from build123d import *

# Parameters (mm, degrees)
SKETCH_1_W          = 45
SKETCH_1_H          = 42
EXTRUDE_1_DEPTH     = 2
SKETCH_2_R          = 11
SKETCH_2_R_2        = 1.5
CUT_EXTRUDE_1_DEPTH = 2
SKETCH_3_W          = 2
SKETCH_3_H          = 42
EXTRUDE_2_DEPTH     = 40
SKETCH_4_R          = 5
SKETCH_4_R_2        = 2.5
EXTRUDE_3_DEPTH     = 10
SKETCH_5_R          = 2
CUT_EXTRUDE_2_DEPTH = 81.950602221


with BuildPart() as part:
    # 草图1 → 凸台-拉伸1 (new body)
    with BuildSketch(Plane(origin=(0, 0, 0), x_dir=(1, 0, 0), z_dir=(0, 1, 0))):
        with Locations((22.5, 21)):
            Rectangle(SKETCH_1_W, SKETCH_1_H)
    extrude(amount=EXTRUDE_1_DEPTH)

    # 草图2 → 切除-拉伸1 (cut)
    with BuildSketch(Plane(origin=(0, 2, 0), x_dir=(1, 0, 0), z_dir=(0, 1, 0))):
        with Locations(Location((21, 21, 0), (0, 0, 270))):
            Circle(SKETCH_2_R)
        with Locations(Location((5.5, 5.5, 0), (0, 0, 270))):
            Circle(SKETCH_2_R_2)
        with Locations(Location((5.5, 36.5, 0), (0, 0, 270))):
            Circle(SKETCH_2_R_2)
        with Locations(Location((36.5, 36.5, 0), (0, 0, 270))):
            Circle(SKETCH_2_R_2)
        with Locations(Location((36.5, 5.5, 0), (0, 0, 270))):
            Circle(SKETCH_2_R_2)
    extrude(amount=-CUT_EXTRUDE_1_DEPTH, mode=Mode.SUBTRACT)

    # 草图3 → 凸台-拉伸2 (add)
    with BuildSketch(Plane(origin=(0, 2, 0), x_dir=(1, 0, 0), z_dir=(0, 1, 0))):
        with Locations((44, 21)):
            Rectangle(SKETCH_3_W, SKETCH_3_H)
    extrude(amount=EXTRUDE_2_DEPTH)

    # 草图4 → 凸台-拉伸3 (add)
    with BuildSketch(Plane(origin=(45, 0, 0), x_dir=(0, 0, -1), z_dir=(1, 0, 0))):
        with Locations(Location((21, 20, 0), (0, 0, 180))):
            Circle(SKETCH_4_R)
        with Locations((21, 20)):
            Circle(SKETCH_4_R_2, mode=Mode.SUBTRACT)
    extrude(amount=EXTRUDE_3_DEPTH)

    # 草图5 → 切除-拉伸2 (cut, through all)
    with BuildSketch(Plane.XY):
        with Locations((50, 20)):
            Circle(SKETCH_5_R)
    extrude(amount=-CUT_EXTRUDE_2_DEPTH, mode=Mode.SUBTRACT)


solid = part.part
Input: part model. Units: mm. Frame: model coordinates. A direction names the side the tool comes from. Give positions to 0.01 mm unless a question says otherwise; leave off trailing zeros. Order: outer loops, then holes, each group sorted by start corner. A loop starts at its lowest first (then second) coordinate and runs counter-clockwise, first axis right, second up. Notation, with made-up numbers: (15, -21) -> (65, -21) arc R19 cw to (65, -12) -> close; hole circle Ø8 at (48.25, -10). An arc over 180 degrees is marked (long way). Use one line per item in the form item = value.
1) Section D-D, the plane z = -17.5. Return loops of the section in (x, y).
Response values:
outline = (0, 0) -> (10.57, 0) -> (10.57, 2) -> (0, 2) -> close; (31.43, 0) -> (45, 0) -> (45, 16.43) -> (55, 16.43) -> (55, 23.57) -> (45, 23.57) -> (45, 42) -> (43, 42) -> (43, 2) -> (31.43, 2) -> close; hole circle Ø4 at (50, 20)
2) Section B-B, the plane z = -5.5. Return loops of the section in (x, y).
Response values:
outline = (0, 0) -> (4, 0) -> (4, 2) -> (0, 2) -> close; (7, 0) -> (35, 0) -> (35, 2) -> (7, 2) -> close; (38, 0) -> (45, 0) -> (45, 42) -> (43, 42) -> (43, 2) -> (38, 2) -> close
3) Mould query, pull axis Z, two halves, no side actions, for faces 4 (the flat face through (32, 1, 0)), 5 (the cylindrical face through (50, 23, -25)), 6 (the cylindrical face through (35.6, 1, -37.7)). Classes: pulls with the +Z half, pulls with the -Z half, needs draft (parallel to the pull), parting line crosses it, or undercut.
Response values:
face_4 = pulls with the +Z half
face_5 = parting line crosses it
face_6 = undercut
4) Line query: probe 1 along X at (y, z) = (1.6, -36.5); probe 2 along X at (y, z) = (20, -18); probe 3 along Y at (x, z) = (37.5, -1.5). Output: solid intervals per line, ascending.
Response values:
probe_1 = 0 to 4, 7 to 35, 38 to 45
probe_2 = 43 to 48, 52 to 55
probe_3 = 0 to 2
5) Reachability of faces 1 (the flat face through (45, 20, -21)), 2 (the flat face through (43, 22, -21)), 3 (the flat face through (44, 42, -21)) from +Z, -Z, +X, -X, +Y, -Y: full face, straight path, thin tool, end or side. Return the list, or none.
Response values:
face_1 = +X
face_2 = +Z, -Z, -X, +Y
face_3 = +Z, -Z, +X, -X, +Y
6) Section A-A, the plane y = 20. Return loops of the section in (x, z).
Response values:
outline = (43, -42) -> (45, -42) -> (45, -26) -> (48, -26) -> (48, -23.5) -> (45, -23.5) -> (45, -18.5) -> (48, -18.5) -> (48, -16) -> (45, -16) -> (45, 0) -> (43, 0) -> close; (52, -26) -> (55, -26) -> (55, -23.5) -> (52, -23.5) -> close; (52, -18.5) -> (55, -18.5) -> (55, -16) -> (52, -16) -> close
7) First-contact query: pin 1 Ø2.5 at (x, z) = (5.5, -5.5) entering from +Y; pin 2 Ø12.5 at (y, z) = (15, -24) entering from +X; pin 3 Ø1.5 at (y, z) = (12, -5) entering from +X; pin 4 Ø1 at (x, z) = (37, -37.5) entering from +Y. Flat tips, straight axial feed; report the tip coordinate or a pass-through.
Response values:
pin_1 = through
pin_2 = 55
pin_3 = 45
pin_4 = 2
8) Section C-C, the plane x = 36.5. Return loops of the section in (y, z), and give its area (3 significant figures).
Response values:
outline = (0, -42) -> (2, -42) -> (2, -38) -> (0, -38) -> close; (0, -35) -> (2, -35) -> (2, -7) -> (0, -7) -> close; (0, -4) -> (2, -4) -> (2, 0) -> (0, 0) -> close
area = 72.0 mm^2
